from build123d import *

# Parameters (mm, degrees)
SKETCH_1_R               = 15
DIAMETER30_HEIGHT8_DEPTH = 8
SKETCH_2_W               = 5.263157895
SKETCH_2_H               = 3.228070175
SKETCH_2_H_2             = 3.087719298
SKETCH_2_H_3             = 2.807017544
CHARACTER_DEPTH          = 0.1
SKETCH_3_R               = 13.1
SKETCH_3_R_2             = 12.7
INK_RING_DEPTH           = 0.08


with BuildPart() as part:
    # 草图1 → Diameter30_Height8 (new body)
    with BuildSketch(Plane.XY):
        Circle(SKETCH_1_R)
    extrude(amount=-DIAMETER30_HEIGHT8_DEPTH)

    # 草图2 → Character_相 (add)
    # profile 1 of 2: a face of its own
    with BuildSketch(Plane.XY):
        with BuildLine():
            add(Edge.make_bspline(
                [(7.561403509, 5.043859649), (7.55019112, 4.760584697), (7.527530744, 4.188082503), (7.508340227, 3.319863454), (7.49462205, 2.433550242), (7.492367, 1.83658782), (7.49122807, 1.535087719)],
                knots=[0, 0, 0, 0, 0.969283805, 1.958934606, 2.969145462, 4, 4, 4, 4], degree=3))
            Line((7.49122807, 1.535087719), (7.49122807, -6.394736842))
            add(Edge.make_bspline(
                [(7.49122807, -6.394736842), (7.494373274, -7.020306568), (7.500608133, -8.260397781), (7.541259106, -9.499836795), (7.561403509, -10.114035088)],
                knots=[0, 0, 0, 0, 1.008909215, 2, 2, 2, 2], degree=3))
            Line((7.561403509, -10.114035088), (6.157894737, -10.114035088))
            Line((6.157894737, -10.114035088), (6.157894737, -8.780701754))
            Line((6.157894737, -8.780701754), (0.894736842, -8.780701754))
            Line((0.894736842, -8.780701754), (0.894736842, -10.254385965))
            Line((0.894736842, -10.254385965), (-0.50877193, -10.254385965))
            add(Edge.make_bspline(
                [(-0.50877193, -10.254385965), (-0.497692205, -9.914790058), (-0.476326497, -9.259926631), (-0.456441705, -8.312053821), (-0.44245572, -7.435279895), (-0.439845263, -6.873840554), (-0.438596491, -6.605263158)],
                knots=[0, 0, 0, 0, 1.117081682, 2.154136505, 3.116988825, 4, 4, 4, 4], degree=3))
            Line((-0.438596491, -6.605263158), (-0.438596491, 1.605263158))
            add(Edge.make_bspline(
                [(-0.438596491, 1.605263158), (-0.439728026, 1.905030661), (-0.441958496, 2.495929231), (-0.45560045, 3.368382891), (-0.474798879, 4.214949159), (-0.497552487, 4.770115799), (-0.50877193, 5.043859649)],
                knots=[0, 0, 0, 0, 1.04583296, 2.06153501, 3.044173712, 4, 4, 4, 4], degree=3))
            Line((-0.50877193, 5.043859649), (7.561403509, 5.043859649))
        make_face()
        with Locations((3.52631579, -5.973684211)):
            Rectangle(SKETCH_2_W, SKETCH_2_H, mode=Mode.SUBTRACT)
        with Locations((3.52631579, 2.307017544)):
            Rectangle(SKETCH_2_W, SKETCH_2_H_2, mode=Mode.SUBTRACT)
        with Locations((3.52631579, -1.763157895)):
            Rectangle(SKETCH_2_W, SKETCH_2_H_3, mode=Mode.SUBTRACT)
    # profile 2 of 2: a face of its own
    with BuildSketch(Plane.XY):
        with BuildLine():
            add(Edge.make_bspline(
                [(-5.070175439, 2.236842105), (-5.069643134, 2.466430588), (-5.068622699, 2.906554508), (-5.075570455, 3.53725376), (-5.079714917, 4.10907054), (-5.087055031, 4.62111986), (-5.098673186, 5.0733128), (-5.106736303, 5.466792434), (-5.12325681, 5.801143721), (-5.135036136, 6.004664303), (-5.140350877, 6.096491228)],
                knots=[0, 0, 0, 0, 1.427178642, 2.735918853, 3.920795363, 4.981877593, 5.919216055, 6.732723881, 7.428214742, 8, 8, 8, 8], degree=3))
            Line((-5.140350877, 6.096491228), (-3.596491228, 6.096491228))
            add(Edge.make_bspline(
                [(-3.596491228, 6.096491228), (-3.601779492, 5.999464476), (-3.613344956, 5.787266417), (-3.630069425, 5.441663603), (-3.638095211, 5.041255673), (-3.649732329, 4.586464135), (-3.657106974, 4.077015184), (-3.661264203, 3.512129116), (-3.668208495, 2.892692888), (-3.667194182, 2.461232429), (-3.666666667, 2.236842105)],
                knots=[0, 0, 0, 0, 0.604055621, 1.321073082, 2.150740011, 3.093471638, 4.149178994, 5.317910599, 6.605121521, 8, 8, 8, 8], degree=3))
            add(Edge.make_bspline(
                [(-3.666666667, 2.236842105), (-3.530644111, 2.236328112), (-3.266384763, 2.235329545), (-2.88174296, 2.242348317), (-2.520442081, 2.246480446), (-2.183393026, 2.253960205), (-1.870707533, 2.265624871), (-1.582020196, 2.273807132), (-1.317912922, 2.290824228), (-1.149878443, 2.301807771), (-1.070175439, 2.307017544)],
                knots=[0, 0, 0, 0, 1.256536578, 2.441150545, 3.553740755, 4.59446206, 5.555405596, 6.444361595, 7.262121348, 8, 8, 8, 8], degree=3))
            Line((-1.070175439, 2.307017544), (-1.070175439, 0.973684211))
            add(Edge.make_bspline(
                [(-1.070175439, 0.973684211), (-1.144677854, 0.978928331), (-1.304031085, 0.990144981), (-1.556887974, 1.006935749), (-1.839513589, 1.015234756), (-2.149605268, 1.026721716), (-2.488385884, 1.034270902), (-2.855751381, 1.03840672), (-3.251657288, 1.045376401), (-3.525446035, 1.044375774), (-3.666666667, 1.043859649)],
                knots=[0, 0, 0, 0, 0.689951739, 1.475737907, 2.340680501, 3.301602752, 4.342301003, 5.470871417, 6.695471813, 8, 8, 8, 8], degree=3))
            Line((-3.666666667, 1.043859649), (-3.666666667, -1.622807018))
            add(Edge.make_bspline(
                [(-3.666666667, -1.622807018), (-3.606636203, -1.561535904), (-3.48182972, -1.434150045), (-3.293392102, -1.23182095), (-3.094864807, -1.013455465), (-2.962807273, -0.859869327), (-2.894736842, -0.780701754)],
                knots=[0, 0, 0, 0, 0.900819035, 1.872850031, 2.903538413, 4, 4, 4, 4], degree=3))
            add(Edge.make_bspline(
                [(-2.894736842, -0.780701754), (-2.689573637, -1.00021337), (-2.288105654, -1.429758644), (-1.724253911, -2.085214095), (-1.199061827, -2.727559357), (-0.877018772, -3.163628299), (-0.719298246, -3.377192982)],
                knots=[0, 0, 0, 0, 1.063555414, 2.081189198, 3.060262768, 4, 4, 4, 4], degree=3))
            add(Edge.make_bspline(
                [(-0.719298246, -3.377192982), (-0.794679109, -3.429771468), (-0.958911081, -3.544323996), (-1.205171009, -3.756414434), (-1.484543132, -4.003739185), (-1.672408418, -4.190524428), (-1.771929825, -4.289473684)],
                knots=[0, 0, 0, 0, 0.790186824, 1.721576733, 2.793008042, 4, 4, 4, 4], degree=3))
            add(Edge.make_bspline(
                [(-1.771929825, -4.289473684), (-1.904998341, -4.0700807), (-2.172035646, -3.629810433), (-2.627101337, -3.003052442), (-3.120200979, -2.3973547), (-3.483629338, -2.022250893), (-3.666666667, -1.833333333)],
                knots=[0, 0, 0, 0, 0.989574309, 1.98584356, 2.985588755, 4, 4, 4, 4], degree=3))
            Line((-3.666666667, -1.833333333), (-3.666666667, -7.166666667))
            add(Edge.make_bspline(
                [(-3.666666667, -7.166666667), (-3.66710265, -7.269767462), (-3.668003985, -7.48291384), (-3.66072287, -7.813831844), (-3.656774838, -8.166472041), (-3.648756785, -8.54161481), (-3.637317912, -8.938358747), (-3.628857904, -9.357787252), (-3.611274705, -9.798652569), (-3.601493913, -10.100167122), (-3.596491228, -10.254385965)],
                knots=[0, 0, 0, 0, 0.801096895, 1.65615505, 2.571793352, 3.541398262, 4.571731919, 5.655903347, 6.80104005, 8, 8, 8, 8], degree=3))
            Line((-3.596491228, -10.254385965), (-5.140350877, -10.254385965))
            add(Edge.make_bspline(
                [(-5.140350877, -10.254385965), (-5.135369022, -10.10016635), (-5.125684865, -9.80038102), (-5.107972861, -9.362986873), (-5.099566341, -8.949620037), (-5.088128806, -8.560674404), (-5.080093207, -8.195928707), (-5.076127742, -7.855416847), (-5.068855811, -7.538361954), (-5.069746959, -7.334744801), (-5.070175439, -7.236842105)],
                knots=[0, 0, 0, 0, 1.22682853, 2.384814657, 3.480414063, 4.514038807, 5.478633795, 6.38111711, 7.221612736, 8, 8, 8, 8], degree=3))
            Line((-5.070175439, -7.236842105), (-5.070175439, -2.464912281))
            add(Edge.make_bspline(
                [(-5.070175439, -2.464912281), (-5.145846519, -2.675980137), (-5.294332566, -3.090149346), (-5.536827031, -3.689408015), (-5.785768752, -4.257890313), (-6.045384746, -4.792645481), (-6.312844256, -5.294903161), (-6.587960306, -5.764116531), (-6.873615691, -6.199513832), (-7.076236773, -6.471903257), (-7.175438596, -6.605263158)],
                knots=[0, 0, 0, 0, 1.153721074, 2.263896326, 3.325849438, 4.34673122, 5.322030602, 6.253316748, 7.144836456, 8, 8, 8, 8], degree=3))
            add(Edge.make_bspline(
                [(-7.175438596, -6.605263158), (-7.255029914, -6.482647166), (-7.407975598, -6.247023641), (-7.657596365, -5.928969858), (-7.897823334, -5.645524257), (-8.073840549, -5.487664221), (-8.157894737, -5.412280702)],
                knots=[0, 0, 0, 0, 1.130515109, 2.172440566, 3.127278412, 4, 4, 4, 4], degree=3))
            add(Edge.make_bspline(
                [(-8.157894737, -5.412280702), (-8.113720781, -5.370641152), (-8.01581978, -5.278357058), (-7.875116797, -5.106371966), (-7.717691149, -4.894771662), (-7.55214221, -4.637411783), (-7.368626266, -4.340225536), (-7.17523642, -3.999537296), (-6.966943261, -3.616722912), (-6.748324508, -3.195711401), (-6.527564492, -2.742508267), (-6.321130463, -2.262276924), (-6.126625974, -1.76162537), (-5.940007338, -1.243020266), (-5.775804486, -0.699655792), (-5.619811727, -0.137450112), (-5.476041057, 0.445727539), (-5.392993233, 0.842595842), (-5.350877193, 1.043859649)],
                knots=[0, 0, 0, 0, 0.40920384, 0.906902363, 1.496106211, 2.188358286, 2.970301714, 3.852632424, 4.830874076, 5.910586812, 7.053030269, 8.231162496, 9.436019769, 10.676532886, 11.948579996, 13.264574909, 14.612783986, 16, 16, 16, 16], degree=3))
            add(Edge.make_bspline(
                [(-5.350877193, 1.043859649), (-5.59606702, 1.042803509), (-6.063956973, 1.040788102), (-6.730227869, 1.027390075), (-7.327421009, 1.009098406), (-7.701367224, 0.985010229), (-7.877192982, 0.973684211)],
                knots=[0, 0, 0, 0, 1.163979785, 2.221195127, 3.163623796, 4, 4, 4, 4], degree=3))
            Line((-7.877192982, 0.973684211), (-7.877192982, 2.307017544))
            add(Edge.make_bspline(
                [(-7.877192982, 2.307017544), (-7.660637158, 2.295769666), (-7.216421348, 2.272697163), (-6.531817674, 2.253723458), (-5.812703734, 2.240131437), (-5.321428092, 2.237955131), (-5.070175439, 2.236842105)],
                knots=[0, 0, 0, 0, 0.926596032, 1.900704393, 2.926359164, 4, 4, 4, 4], degree=3))
        make_face()
    extrude(amount=CHARACTER_DEPTH)

    # 草图3 → Ink_ring (add)
    with BuildSketch(Plane.XY):
        with Locations(Location((0, 0, 0), (0, 0, 180))):
            Circle(SKETCH_3_R)
        with Locations(Location((0, 0, 0), (0, 0, 180))):
            Circle(SKETCH_3_R_2, mode=Mode.SUBTRACT)
    extrude(amount=INK_RING_DEPTH)


solid = part.part
Verification items for the finished model (mm, model axes). A direction names the side the tool comes from. Coordinates: 2 decimals unless noted, no trailing zeros. Order: outer loops, then holes, each group sorted by start corner. A loop starts at its lowest first (then second) coordinate and runs counter-clockwise, first axis right, second up.
Item 1: Section check A-A, the plane z = -4. Enter the section's corners in (x, y), then the cut area to 3 significant figures.
Filled in:
outline: circle Ø30 at (0, 0)
area: 707 mm2
Item 2: Material ranges on L1, parallel to Z at x = 6, y = 3.75; L2, parallel to Y at x = 0.75, z = -0.25; L3, parallel to Y at x = -2.5, z = -2.5, recorded low to high.
Filled in:
L1: z = -8 to 0
L2: y = -14.98 to 14.98
L3: y = -14.79 to 14.79
Item 3: Depth check by flat-ended pin: pin 1 (1 mm diameter, centred on x = -9, y = -8, fed in from +Z); pin 2 (1 mm diameter, centred on x = 10.5, z = -7, fed in from +Y); pin 3 (1.5 mm diameter, centred on x = 9.5, z = -6, fed in from -Y). Enter the tip coordinate at first touch or a pass-through.
Filled in:
pin 1: stops at z = 0
pin 2: stops at y = 11.18
pin 3: stops at y = -12.18
Item 4: Section check B-B, the plane x = 8.75. Enter the section's corners in (y, z), then the cut area to 3 significant figures.
Filled in:
outline: (-12.18, -8) - (12.18, -8) - (12.18, 0) - (9.75, 0) - (9.75, 0.08) - (9.2, 0.08) - (9.2, 0) - (-9.2, 0) - (-9.2, 0.08) - (-9.75, 0.08) - (-9.75, 0) - (-12.18, 0) - close
area: 195 mm2
Item 5: Release check for a two-part mould opening along Y. For faces 3 (the face through (-14.985, 0.66, -3.944)), 4 (the face through (3, -6, 0)), 5 (the face through (-5, -1, 0.1)) record: +Y half, -Y half, draft (parallel to the pull), parting line (faces both ways), or undercut.
Filled in:
face 3: parting line
face 4: undercut
face 5: draft
Item 6: Access from +Z, -Z, +X, -X, +Y, -Y to the whole of each face (thin tool, end or side, straight path). Record for faces 1 (the face through (0, 0, -8)), 2 (the face through (3, 2, 0)).
Filled in:
face 1: -Z, +X, -X, +Y, -Y
face 2: +Z
